Could you check a few things on this model? Use its own coordinates, in mm. Face numbers are marked on the shaded views. Give positions to 0.01 mm unless a question says otherwise; leave off trailing zeros. Write each loop counter-clockwise with the first axis right and the second up, starting at its lowest first coordinate (ties: lowest second). Pieces come first, ordered by that corner, then holes. Notation, with made-up numbers: (-24.75, 46.25) -> (20.25, 46.25) arc R20 ccw to (20.25, 61.25) -> close; hole circle Ø4 at (47, 3.25). An arc over 180 degrees is marked (long way). One line per question, with ' | ' between items.
from build123d import *

# Parameters (mm, degrees)
F0_W         = 46
F0_H         = 11
F1_DEPTH     = 180
F2_T         = -2.5
F3_T1_DEPTH  = 71
F4_R         = 5
F5_T1_DEPTH  = 187.5
F5_T3_DEPTH  = 1
F5_T6_ANGLE  = 90
F5_T8_ANGLE  = 89.9999999974
F5_T10_ANGLE = 90
F5_T12_ANGLE = 89.9999999974


# Not quite as in the source:
# - a fillet or chamfer that OpenCascade refuses, or shapes differently, is made with other operations: its cross-section is extruded or revolved along the edge and cut away or added


with BuildPart() as f1:
    # F0 (on Top) → F1 (new body)
    with BuildSketch(Plane.XY):
        with Locations((23, -5.5)):
            Rectangle(F0_W, F0_H)
    extrude(amount=F1_DEPTH)

    # F2
    f2_openings = [f1.faces().sort_by_distance(p)[0] for p in [
        (23, 0, 90),
    ]]
    offset(amount=F2_T, openings=f2_openings)

    # F3: fillet of radius 5 on 1 edges, made by hand

    # F3_s2 → F3_t1 (cut)
    with BuildSketch(Plane.YZ.offset(-12.5)):
        with BuildLine():
            ThreePointArc((-5, 0), (-1.4644660941, 1.4644660941), (0, 5))
            Line((0, 5), (0, 0))
            Line((0, 0), (-5, 0))
        make_face()
    extrude(amount=F3_T1_DEPTH, mode=Mode.SUBTRACT)

    # F4
    f4_edges = [f1.edges().sort_by_distance(p)[0] for p in [
        (23, -11, 0),
    ]]
    fillet(f4_edges, radius=F4_R)

    # F5: fillet of radius 5 on 2 edges, made by hand

    # F5_s2 → F5_t1 (cut)
    with BuildSketch(Plane.XY.offset(5)):
        with BuildLine():
            ThreePointArc((0, -6), (1.4644660941, -9.5355339059), (5, -11))
            Line((5, -11), (0, -11))
            Line((0, -11), (0, -6))
        make_face()
        with BuildLine():
            ThreePointArc((41, -11), (44.5355339059, -9.5355339059), (46, -6))
            Line((46, -6), (46, -11))
            Line((46, -11), (41, -11))
        make_face()
        with BuildLine():
            ThreePointArc((41, 0), (44.5355339059, -1.4644660941), (46, -5))
            Line((46, -5), (46, 0))
            Line((46, 0), (41, 0))
        make_face()
        with BuildLine():
            ThreePointArc((0, -5), (1.4644660941, -1.4644660941), (5, 0))
            Line((5, 0), (0, 0))
            Line((0, 0), (0, -5))
        make_face()
    extrude(amount=F5_T1_DEPTH, mode=Mode.SUBTRACT)

    # F5_s4 → F5_t3 (cut)
    with BuildSketch(Plane.XZ.offset(5)):
        with BuildLine():
            ThreePointArc((41, 0), (44.5355339059, 1.4644660941), (46, 5))
            Line((46, 5), (46, 0))
            Line((46, 0), (41, 0))
        make_face()
        with BuildLine():
            ThreePointArc((0, 5), (1.4644660941, 1.4644660941), (5, 0))
            Line((5, 0), (0, 0))
            Line((0, 0), (0, 5))
        make_face()
    extrude(amount=F5_T3_DEPTH, mode=Mode.SUBTRACT)

    # F5_s5 → F5_t6 (revolve, cut)
    with BuildSketch(Plane.XZ.offset(6)):
        with BuildLine():
            ThreePointArc((41, 0), (44.5355339059, 1.4644660941), (46, 5))
            Line((46, 5), (46, 0))
            Line((46, 0), (41, 0))
        make_face()
    revolve(axis=Axis((46, -6, 5), (-1, 0, 0)), revolution_arc=F5_T6_ANGLE, mode=Mode.SUBTRACT)

    # F5_s7 → F5_t8 (revolve, cut)
    with BuildSketch(Plane.XY.offset(5.0000000001)):
        with BuildLine():
            ThreePointArc((41, 0), (44.5355339059, -1.4644660941), (46, -5))
            Line((46, -5), (46, 0))
            Line((46, 0), (41, 0))
        make_face()
    revolve(axis=Axis((46, -5.0000000001, 5.0000000001), (-1, 0, 0)), revolution_arc=F5_T8_ANGLE, mode=Mode.SUBTRACT)

    # F5_s9 → F5_t10 (revolve, cut)
    with BuildSketch(Plane.XZ.offset(6)):
        with BuildLine():
            ThreePointArc((0, 5), (1.4644660941, 1.4644660941), (5, 0))
            Line((5, 0), (0, 0))
            Line((0, 0), (0, 5))
        make_face()
    revolve(axis=Axis((0, -6, 5), (-1, 0, 0)), revolution_arc=F5_T10_ANGLE, mode=Mode.SUBTRACT)

    # F5_s11 → F5_t12 (revolve, cut)
    with BuildSketch(Plane.XY.offset(5.0000000001)):
        with BuildLine():
            ThreePointArc((0, -5), (1.4644660941, -1.4644660941), (5, 0))
            Line((5, 0), (0, 0))
            Line((0, 0), (0, -5))
        make_face()
    revolve(axis=Axis((0, -5.0000000001, 5.0000000001), (-1, 0, 0)), revolution_arc=F5_T12_ANGLE, mode=Mode.SUBTRACT)


solid = f1.part
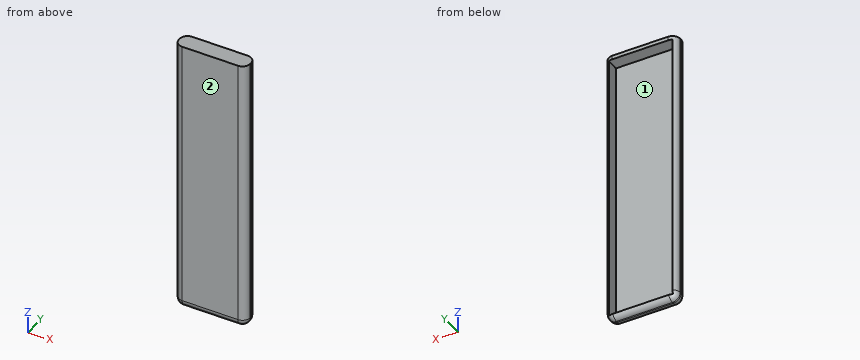
Q1. If I drill on line 1 along Z through (x, y) = (17.5, -5.5); line 2 along X through (y, z) = (-5, 154.5); line 3 along Y through (x, z) = (33, 13), over which ranges is the centre line in solid material (lowest first)?
Answer below:
line 1: z = 0 to 2.5, 177.5 to 180 | line 2: x = 0 to 2.5, 43.5 to 46 | line 3: y = -11 to -8.5
Q2. Will these pins go through, and if not, where does the flat tip stop? pin 1 (1 mm diameter, centred on y = -9.5, z = 138.5, fed in from +X); pin 2 (20.5 mm diameter, centred on x = 14.5, z = 82, fed in from +Y); pin 3 (2.5 mm diameter, centred on x = 20.5, y = -3.5, fed in from -Z).
Answer below:
pin 1: stops at x = 45 | pin 2: stops at y = -8.5 | pin 3: stops at z = 0.01
Q3. Imagine slicing it at B-B on x = 22. Please give me the cut outline in (y, z).
Answer below:
outline: (-11, 5) arc R5 ccw to (-6, 0) -> (-5, 0) arc R5 ccw to (-0.67, 2.5) -> (-8.5, 2.5) -> (-8.5, 177.5) -> (0, 177.5) -> (0, 180) -> (-11, 180) -> close
Q4. Imagine slicing it at C-C on y = -3.5. Please give me the cut outline in (x, z), and give its area (3 significant figures).
Answer below:
outline: (0.23, 5) arc R4.77 ccw to (5, 0.23) -> (41, 0.23) arc R4.77 ccw to (45.77, 5) -> (45.77, 180) -> (0.23, 180) -> close; hole (2.5, 2.5) -> (43.5, 2.5) -> (43.5, 177.5) -> (2.5, 177.5) -> close | area: 1,000 mm^2
Q5. If we mould it in two halves opening along Z, with no side actions, what happens to the marked faces 1 and 2? For each: +Z half, -Z half, draft (parallel to the pull), parting line (faces both ways), or undercut.
Answer below:
face 1: undercut | face 2: draft
Q6. Imagine slicing it at A-A on z = 66. Please give me the cut outline in (x, y).
Answer below:
outline: (0, -6) arc R5 ccw to (5, -11) -> (41, -11) arc R5 ccw to (46, -6) -> (46, -5) arc R5 ccw to (43.5, -0.67) -> (43.5, -8.5) -> (2.5, -8.5) -> (2.5, -0.67) arc R5 ccw to (0, -5) -> close
